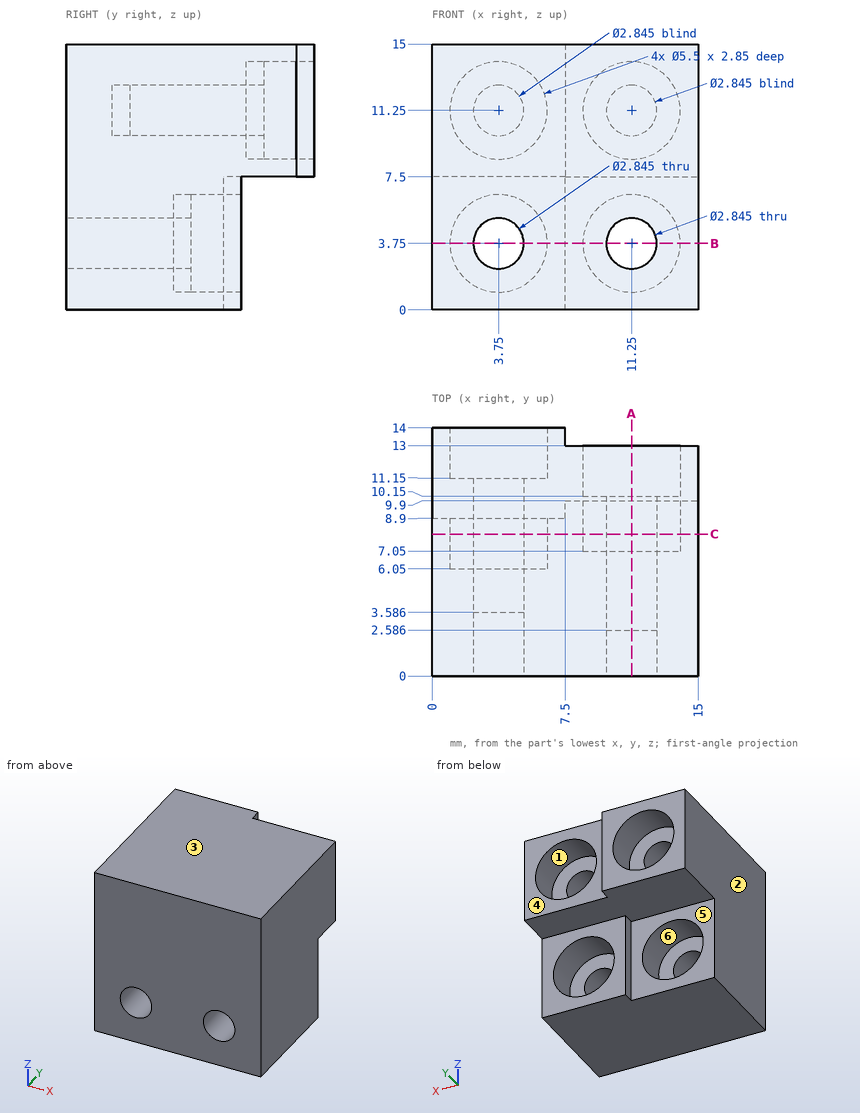
The figure shows three views and two pictorial views of one solid part (mm, origin at its lowest corner). Answer the questions. A direction names the side the tool comes from. Coordinates: 2 decimals unless noted, no trailing zeros. Loops run counter-clockwise (first coordinate to the right, second up) from the corner with the lowest first, then second, coordinate; pieces in that order, holes last. Notation, with made-up numbers: (1, -9) -> (56, -9) arc R20 ccw to (56, 20) -> close; hole circle Ø4 at (-16.5, -33.5). An arc over 180 degrees is marked (long way). Return JSON: item names as keys, results as strings. Group by question number.
(1) Determine the mould class of the marked faces 1, 2 and 3 for opening direction X: released by +X, released by -X, zero draft, split by the parting line, or undercut.
(2) Given pin 1 Ø8 at (x, z) = (12.5, 4.5) entering from +Y; pin 2 Ø6 at (x, z) = (4, 4) entering from +Y; pin 3 Ø0.8 at (y, z) = (13.5, 11.5) entering from +X; pin 4 Ø3.5 at (x, z) = (11.25, 3.75) entering from -Y, each flat-ended and moving along its own axis, determine where each tip first touches the part or whether it passes through.
(3) A cutting plane is placed at A-A on x = 11.25. Write down the section's boundary in (y, z).
(4) Which of the six approach directions +Z, -Z, +X, -X, +Y, -Y give full straight-line access (tool end or side, diameter ignored) to the marked faces 4, 5 and 6?
(5) A cutting plane is placed at C-C on y = 8. Count the separate pieces of the cut face and the enclosed holes in it, and give its area (3 significant figures).
(6) A cutting plane is placed at B-B on z = 3.75. Write down the section's boundary in (x, y), and give its area (3 significant figures).
(7) Find the intervals of material crossed by probe 1 along Z at (x, y) = (11.25, 8.5); probe 2 along X at (y, z) = (7.8, 3.75); probe 3 along Z at (x, y) = (11.25, 3.5), in increasing order. Write a range as from..to.
The answers:
{
 "1": {"face 1": "undercut", "face 2": "released by -X", "face 3": "zero draft"},
 "2": {"pin 1": "stops at y = 13", "pin 2": "stops at y = 8.9", "pin 3": "stops at x = 7.5", "pin 4": "stops at y = 0"},
 "3": {"outline": "(0, 0) -> (9.9, 0) -> (9.9, 1) -> (7.05, 1) -> (7.05, 2.33) -> (0, 2.33) -> close; (0, 5.17) -> (7.05, 5.17) -> (7.05, 6.5) -> (9.9, 6.5) -> (9.9, 7.5) -> (13, 7.5) -> (13, 8.5) -> (10.15, 8.5) -> (10.15, 9.83) -> (2.59, 9.83) -> (2.59, 12.67) -> (10.15, 12.67) -> (10.15, 14) -> (13, 14) -> (13, 15) -> (0, 15) -> close"},
 "4": {"face 4": "+Z, -Z, +X, +Y", "face 5": "-Z, -X, +Y", "face 6": "+Y"},
 "5": {"separate pieces": "1", "enclosed holes": "4", "area": "165 mm^2"},
 "6": {"outline": "(0, 0) -> (2.33, 0) -> (2.33, 6.05) -> (1, 6.05) -> (1, 8.9) -> (0, 8.9) -> close; (5.17, 0) -> (9.83, 0) -> (9.83, 7.05) -> (8.5, 7.05) -> (8.5, 9.9) -> (7.5, 9.9) -> (7.5, 8.9) -> (6.5, 8.9) -> (6.5, 6.05) -> (5.17, 6.05) -> close; (12.67, 0) -> (15, 0) -> (15, 9.9) -> (14, 9.9) -> (14, 7.05) -> (12.67, 7.05) -> close", "area": "72.4 mm^2"},
 "7": {"probe 1": "z = 0..1, 6.5..9.83, 12.67..15", "probe 2": "x = 0..1, 6.5..8.5, 14..15", "probe 3": "z = 0..2.33, 5.17..9.83, 12.67..15"}
}
